Geometry: final body of the model. Coordinates: model frame, mm. Face numbers are marked on the shaded views. A direction names the side the tool comes from. Round coordinates to 2 decimals unless told otherwise and drop trailing zeros. Loops run counter-clockwise (first coordinate to the right, second up) from the corner with the lowest first, then second, coordinate; pieces in that order, holes last. Notation, with made-up numbers: (75.25, 4) - (94.25, 4) arc R27 cw to (94.25, 31) - close; hole circle Ø5 at (36, 13). An arc over 180 degrees is marked (long way). Answer as a JSON object with one key per item and string values. Group by question number.
Item 1: Section C-C (y = 12.5). Count the separate pieces of the cut face and the enclosed holes in it, plus the area to 3 significant figures.
Item 2: Draft query along Y for the marked faces 3, 4 and 5. Return one class per face: released by +Y, released by -Y, zero draft, split by the parting line, or undercut.
Item 3: Section A-A (z = 13). Return the cut outline in (x, y) (3 decimals).
Item 4: Reachability of the marked faces 1 and 2 from +Z, -Z, +X, -X, +Y, -Y: full face, straight path, thin tool, end or side. Return the list, or none.
Item 5: First-contact query: pin 1 (6 mm diameter, centred on x = -5, z = 6, fed in from -Y); pin 2 (8 mm diameter, centred on x = 23.5, z = 9, fed in from -Y); pin 3 (2 mm diameter, centred on x = -6, z = 5.5, fed in from +Y); pin 4 (4 mm diameter, centred on x = 0, y = 40, fed in from -Z). Flat tips, straight axial feed; report the tip coordinate or a pass-through.
Item 6: Line query: line 1 (Z direction, x = 29, y = -25.5); line 2 (Y direction, x = -7, z = 5.5); line 3 (X direction, y = 5.5, z = 12). Output: solid intervals per line, ascending.
Item 7: Section B-B (x = 0). Return the cut outline in (y, z), plus the area to 3 significant figures.
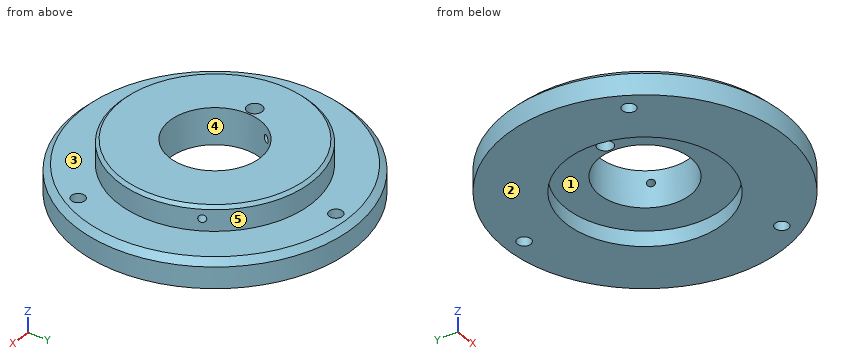
```python
from build123d import *

# Parameters (mm, degrees)
ESQUISSE1_R                  = 46
BASE_EXTRUSION_DEPTH         = 9
ESQUISSE2_R                  = 32
BOSS_EXTRU_1_DEPTH           = 8
ESQUISSE3_R                  = 26
ENL_V_MAT_EXTRU_1_DEPTH      = 5
ESQUISSE4_R                  = 15
ENL_V_MAT_EXTRU_2_DEPTH      = 13
ESQUISSE5_R                  = 2.2
ENL_V_MAT_EXTRU_3_DEPTH      = 10
R_P_TITION_CIRCULAIRE1_COUNT = 3
CHANFREIN1_SIZE              = 2
CHANFREIN2_SIZE              = 1
ENL_V_START                  = -17.050105
ESQUISSE8_R                  = 1.225
ENL_V_MAT_EXTRU_4_DEPTH      = 17.050105
R_P_TITION_CIRCULAIRE2_COUNT = 2
R_P_TITION_CIRCULAIRE2_ANGLE = 120
ESQUISSE9_R                  = 2.5
ENL_V_MAT_EXTRU_5_DEPTH      = 18


with BuildPart() as part:
    # Esquisse1 → Base-Extrusion (new body)
    with BuildSketch(Plane.XY):
        Circle(ESQUISSE1_R)
    extrude(amount=BASE_EXTRUSION_DEPTH)

    # Esquisse2 → Boss.-Extru.1 (add)
    with BuildSketch(Plane.XY.offset(9)):
        Circle(ESQUISSE2_R)
    extrude(amount=BOSS_EXTRU_1_DEPTH)

    # Esquisse3 → Enlèv. mat.-Extru.1 (cut)
    with BuildSketch(Plane(origin=(0, 0, 0), x_dir=(-1, 0, 0), z_dir=(0, 0, -1))):
        Circle(ESQUISSE3_R)
    extrude(amount=-ENL_V_MAT_EXTRU_1_DEPTH, mode=Mode.SUBTRACT)

    # Esquisse4 → Enlèv. mat.-Extru.2 (cut, through all)
    with BuildSketch(Plane(origin=(0, 0, 5), x_dir=(-1, 0, 0), z_dir=(0, 0, -1))):
        Circle(ESQUISSE4_R)
    extrude(amount=-ENL_V_MAT_EXTRU_2_DEPTH, mode=Mode.SUBTRACT)

    # Esquisse5 → Enlèv. mat.-Extru.3 (cut, through all)
    with BuildSketch(Plane.XY.offset(9)):
        with Locations((0, 40)):
            Circle(ESQUISSE5_R)
    enl_v_mat_extru_3 = extrude(amount=-ENL_V_MAT_EXTRU_3_DEPTH, mode=Mode.SUBTRACT)

    # Répétition circulaire1: Enlèv. mat.-Extru.3 ×3 about axis
    r_p_tition_circulaire1_axis = Axis((0, 0, 0), (0, 0, 1))
    for i in range(1, R_P_TITION_CIRCULAIRE1_COUNT):
        add(enl_v_mat_extru_3.rotate(r_p_tition_circulaire1_axis, i * 360 / R_P_TITION_CIRCULAIRE1_COUNT), mode=Mode.SUBTRACT)

    # Chanfrein1
    chanfrein1_edges = [part.edges().sort_by_distance(p)[0] for p in [
        (-46, 0, 9),
    ]]
    chamfer(chanfrein1_edges, length=CHANFREIN1_SIZE)

    # Chanfrein2
    chanfrein2_edges = [part.edges().sort_by_distance(p)[0] for p in [
        (-32, 0, 17),
    ]]
    chamfer(chanfrein2_edges, length=CHANFREIN2_SIZE)

    # Esquisse8 → Enlèv. mat.-Extru.4 (cut)
    with BuildSketch(Plane(origin=(27.712812921, 16, 0), x_dir=(0, 0, -1), z_dir=(0.866025404, 0.5, 0)).offset(ENL_V_START)):
        with Locations((-13, 0)):
            Circle(ESQUISSE8_R)
    enl_v_mat_extru_4 = extrude(amount=ENL_V_MAT_EXTRU_4_DEPTH, mode=Mode.SUBTRACT)

    # Répétition circulaire2: Enlèv. mat.-Extru.4 ×2 about axis
    r_p_tition_circulaire2_axis = Axis((0, 0, 17), (0, 0, 1))
    for i in range(1, R_P_TITION_CIRCULAIRE2_COUNT):
        add(enl_v_mat_extru_4.rotate(r_p_tition_circulaire2_axis, i * R_P_TITION_CIRCULAIRE2_ANGLE / (R_P_TITION_CIRCULAIRE2_COUNT - 1)), mode=Mode.SUBTRACT)

    # Esquisse9 → Enlèv. mat.-Extru.5 (cut, through all)
    with BuildSketch(Plane.XY.offset(17)):
        with Locations((-18, 0)):
            Circle(ESQUISSE9_R)
    extrude(amount=-ENL_V_MAT_EXTRU_5_DEPTH, mode=Mode.SUBTRACT)


solid = part.part
```
Values:
{
 "1": {"separate pieces": "2", "enclosed holes": "2", "area": "817 mm^2"},
 "2": {"face 3": "zero draft", "face 4": "undercut", "face 5": "split by the parting line"},
 "3": {"outline": "(-28.305, 14.927) arc R32 ccw (long way) to (28.305, 14.927) - (13.559, 6.414) arc R15 cw (long way) to (-13.559, 6.414) - close; (-27.08, 17.049) - (-12.334, 8.536) arc R15 cw to (12.334, 8.536) - (27.08, 17.049) arc R32 ccw to start; hole circle Ø5 at (-18, 0)"},
 "4": {"face 1": "-Z", "face 2": "-Z, +X, -X, +Y, -Y"},
 "5": {"pin 1": "stops at y = -45.96", "pin 2": "stops at y = -41.41", "pin 3": "stops at y = 45.73", "pin 4": "passes through"},
 "6": {"line 1": "z = 0 to 9", "line 2": "y = -45.46 to -13.27, 13.27 to 45.46", "line 3": "x = -31.52 to -13.96, 13.96 to 31.52"},
 "7": {"outline": "(-46, 0) - (-26, 0) - (-26, 5) - (-15, 5) - (-15, 17) - (-31, 17) - (-32, 16) - (-32, 9) - (-44, 9) - (-46, 7) - close; (15, 5) - (26, 5) - (26, 0) - (37.8, 0) - (37.8, 9) - (32, 9) - (32, 16) - (31, 17) - (15, 17) - close; (42.2, 0) - (46, 0) - (46, 7) - (44, 9) - (42.2, 9) - close", "area": "675 mm^2"}
}
